The figure shows three views and two pictorial views of one solid part (mm, origin at its lowest corner). Answer the questions. A direction names the side the tool comes from. Round coordinates to 2 decimals unless told otherwise and drop trailing zeros. Write each loop counter-clockwise with the first axis right and the second up, starting at its lowest first coordinate (ties: lowest second). Pieces come first, ordered by that corner, then holes. Notation, with made-up numbers: (65, -8) -> (73, -8) arc R9 ccw to (73, 6) -> close; hole circle Ø2 at (73.5, 67). An arc over 180 degrees is marked (long way). One line per item, written item: value.
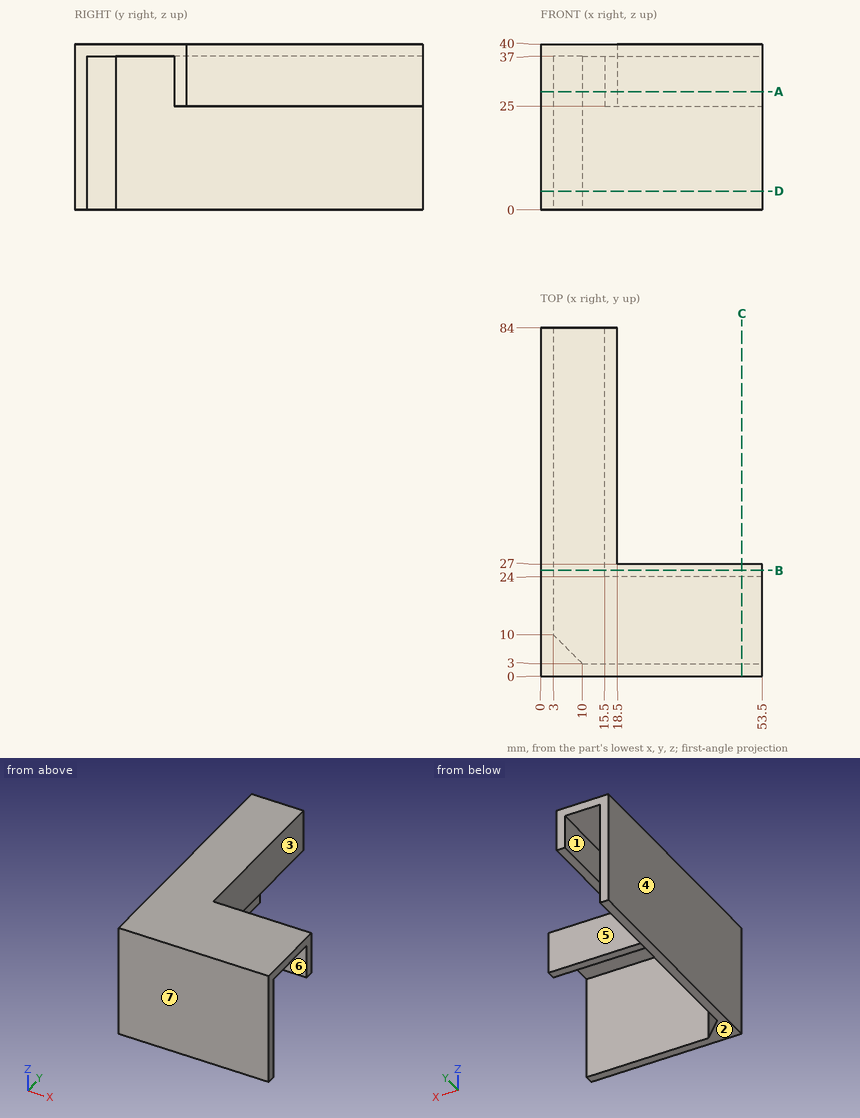
(1) A tool of negligible diameter and unlimited length cuts with its end or side. For the marked faces 5, 6 and 7, from which of +Z, -Z, +X, -X, +Y, -Y can it reach the whole face along a straight path? Write none if from no direction.
Reported:
face 5: +Z, -Z, +X, +Y
face 6: -Z, +X
face 7: +Z, -Z, +X, -X, -Y
(2) For a pull along X with two mould halves and no side action, classify the marked faces 1, 2, 3 and 4 as pulls with the +X half, pulls with the -X half, needs draft (parallel to the pull), parting line crosses it, or undercut.
Reported:
face 1: undercut
face 2: needs draft
face 3: pulls with the +X half
face 4: pulls with the -X half
(3) Find section A-A on z = 28.5. Give the vertices of the cut face in (x, y).
Reported:
outline: (0, 0) -> (53.5, 0) -> (53.5, 3) -> (10, 3) -> (3, 10) -> (3, 84) -> (0, 84) -> close; (15.5, 24) -> (53.5, 24) -> (53.5, 27) -> (18.5, 27) -> (18.5, 84) -> (15.5, 84) -> close
(4) Find section D-D on z = 4.5. Give the vertices of the cut face in (x, y), plus the area to 3 significant figures.
Reported:
outline: (0, 0) -> (53.5, 0) -> (53.5, 3) -> (10, 3) -> (3, 10) -> (3, 84) -> (0, 84) -> close
area: 428 mm2
(5) Consider probe 1 along X at (y, z) = (45.5, 26); probe 2 along Y at (x, z) = (40.5, 34); probe 3 along Y at (x, z) = (36, 7.5). Determine where each line is inside the solid, lowest interval first.
Reported:
probe 1: x = 0 to 3, 15.5 to 18.5
probe 2: y = 0 to 3, 24 to 27
probe 3: y = 0 to 3
(6) Find section C-C on x = 48.5. Give the vertices of the cut face in (y, z), plus the area to 3 significant figures.
Reported:
outline: (0, 0) -> (3, 0) -> (3, 37) -> (24, 37) -> (24, 25) -> (27, 25) -> (27, 40) -> (0, 40) -> close
area: 228 mm2
(7) Find section B-B on y = 25.5. Give the vertices of the cut face in (x, z).
Reported:
outline: (0, 0) -> (3, 0) -> (3, 37) -> (15.5, 37) -> (15.5, 25) -> (53.5, 25) -> (53.5, 40) -> (0, 40) -> close
(8) Flat-ended cylindrical pins translate along their axes: pin 1 Ø3 at (x, y) = (33, 19) entering from -Z; pin 2 Ø4.5 at (x, z) = (36.5, 34) entering from +Y; pin 3 Ø16.5 at (y, z) = (59, 35.5) entering from +X. Find the tip coordinate at first contact, or state that the pin passes through.
Reported:
pin 1: stops at z = 37
pin 2: stops at y = 27
pin 3: stops at x = 18.5
